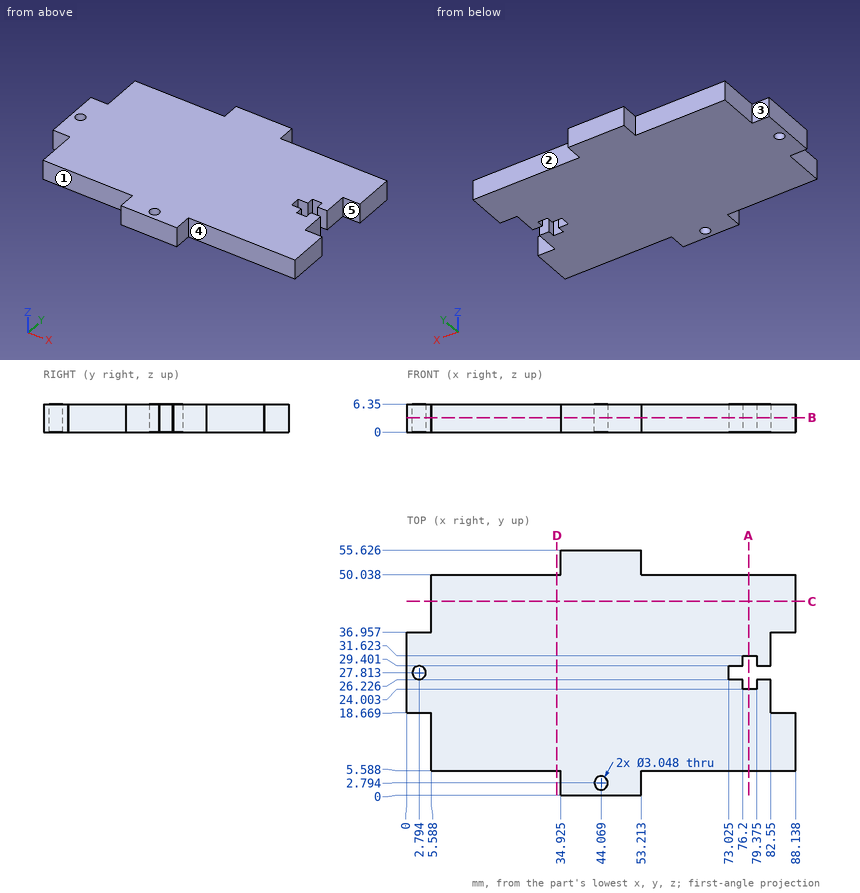
Source: three-view drawing plus pictorial views. Frame: mm from the lowest corner of the part. A direction names the side the tool comes from. Round coordinates to 2 decimals unless told otherwise and drop trailing zeros. Loops run counter-clockwise (first coordinate to the right, second up) from the corner with the lowest first, then second, coordinate; pieces in that order, holes last.
Q1. Section B-B on z = 3.25. State how many separate pieces and enclosed holes the cut face has.
Q2. Material intervals for L1, parallel to X at y = 28, z = 4.25 (1 decimal); L2, parallel to Y at x = 70, z = 0.75; L3, parallel to X at y = 23.5, z = 5, sorted ascending.
Q3. Section C-C on y = 44. Return loops of the section in (x, z).
Q4. Pin query (flat end, axial travel): P1, Ø1.9, axis at y = 43, z = 4, coming from the -X side; P2, Ø1, axis at x = 80.5, z = 2, coming from the +Y side; P3, Ø1, axis at x = 81.5, z = 4.5, coming from the -Y side. Return the tip coordinate at first contact, or that it passes through.
Q5. Section A-A on x = 77.5. Return loops of the section in (y, z), plus the area to 3 significant figures.
Q6. Section D-D on x = 34. Return loops of the section in (y, z), plus the area to 3 significant figures.
Q7. Access query for the marked faces 1, 2, 3, 4 and 5. Directions: +Z, -Z, +X, -X, +Y, -Y. A direction counts if a zero-diameter tool reaches every point of the face in a straight line with its end or side. Return the directions, or none.
Evaluation:
1. separate pieces: 1
1. enclosed holes: 2
2. L1: x = 0 to 1.3, 4.3 to 73
2. L2: y = 5.59 to 50.04
2. L3: x = 0 to 82.55
3. outline: (5.59, 0) - (88.14, 0) - (88.14, 6.35) - (5.59, 6.35) - close
4. P1: stops at x = 5.59
4. P2: stops at y = 50.04
4. P3: stops at y = 5.59
5. outline: (5.59, 0) - (24, 0) - (24, 6.35) - (5.59, 6.35) - close; (31.62, 0) - (50.04, 0) - (50.04, 6.35) - (31.62, 6.35) - close
5. area: 234 mm2
6. outline: (5.59, 0) - (50.04, 0) - (50.04, 6.35) - (5.59, 6.35) - close
6. area: 282 mm2
7. face 1: +Z, -Z, -X, -Y
7. face 2: +Z, -Z, +X, +Y
7. face 3: +Z, -Z, -X, +Y
7. face 4: +Z, -Z, +X, -Y
7. face 5: +Z, -Z, +X
